from build123d import *

# Parameters (mm, degrees)
F0_R     = 4.05
F1_DEPTH = 1.5
F2_R     = 1
F3_DEPTH = 12.5


with BuildPart() as f1:
    # F0 (on Front) → F1 (new body, symmetric)
    with BuildSketch(Plane.XZ):
        with BuildLine():
            Line((0.714422, -9.773925), (32.096751, -7.480044))
            ThreePointArc((32.096751, -7.480044), (39.05, 0), (32.096751, 7.480044))
            Line((32.096751, 7.480044), (0.714422, 9.773925))
            ThreePointArc((0.714422, 9.773925), (-9.8, 0), (0.714422, -9.773925))
        make_face()
        Circle(F0_R, mode=Mode.SUBTRACT)
        with BuildLine():
            ThreePointArc((32, 0.95), (32.95, 0), (32, -0.95))
            Line((32, -0.95), (7, -0.95))
            ThreePointArc((7, -0.95), (6.05, 0), (7, 0.95))
            Line((7, 0.95), (32, 0.95))
        make_face(mode=Mode.SUBTRACT)
    extrude(amount=F1_DEPTH, both=True)

    # F2 (on Top) → F3 (cut, symmetric)
    with BuildSketch(Plane.XY):
        Circle(F2_R)
    extrude(amount=F3_DEPTH, both=True, mode=Mode.SUBTRACT)


solid = f1.part
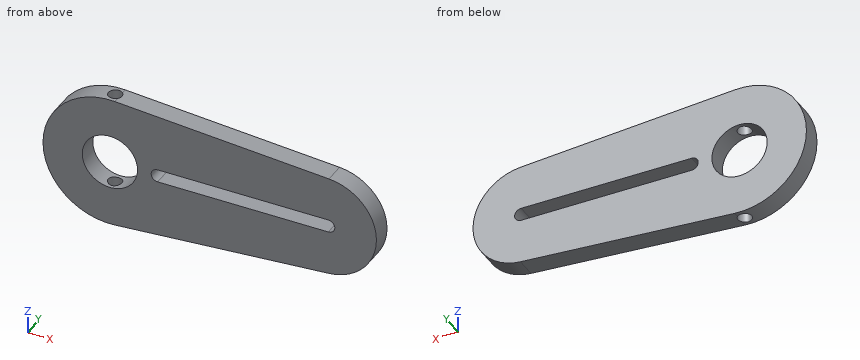
Geometry check sheet. Reference: the model listing, model coordinates, mm. Round coordinates to 2 decimals unless told otherwise and drop trailing zeros. Write each loop counter-clockwise with the first axis right and the second up, starting at its lowest first coordinate (ties: lowest second). Pieces come first, ordered by that corner, then holes.
Item 1: Section check A-A (x = 0). Record the boundary of the cut face in (y, z).
Determined:
outline: (-1.5, -9.8) - (-1, -9.8) - (-1, -4.05) - (-1.5, -4.05) - close; (-1.5, 4.05) - (-1, 4.05) - (-1, 9.8) - (-1.5, 9.8) - close; (1, -9.8) - (1.5, -9.8) - (1.5, -4.05) - (1, -4.05) - close; (1, 4.05) - (1.5, 4.05) - (1.5, 9.8) - (1, 9.8) - close
Item 2: Go/stop test with flat-tipped pins: pin 1 Ø1.2 at (x, y) = (0, 0) entering from -Z; pin 2 Ø1.5 at (x, y) = (29.5, 1) entering from +Z; pin 3 Ø1.5 at (x, y) = (15, 0.5) entering from -Z. Record where each tip stops, or that it passes through.
Determined:
pin 1: passes through
pin 2: stops at z = 7.72
pin 3: stops at z = -8.78
Item 3: Section check D-D (x = 10). Record the boundary of the cut face in (y, z).
Determined:
outline: (-1.5, -9.1) - (1.5, -9.1) - (1.5, -0.95) - (-1.5, -0.95) - close; (-1.5, 0.95) - (1.5, 0.95) - (1.5, 9.1) - (-1.5, 9.1) - close
Item 4: Section check C-C (y = 0). Record the boundary of the cut face in (x, z), plus the area to 3 significant figures.
Determined:
outline: (-1, -9.75) - (-1, -3.92) arc R4.05 cw to (-1, 3.92) - (-1, 9.75) arc R9.8 ccw to start; (1, -9.75) - (32.1, -7.48) arc R7.5 ccw to (32.1, 7.48) - (1, 9.75) - (1, 3.92) arc R4.05 cw to (1, -3.92) - close; hole (7, -0.95) - (32, -0.95) arc R0.95 ccw to (32, 0.95) - (7, 0.95) arc R0.95 ccw to start
area: 662 mm2
Item 5: Section check B-B (z = 0). Record the boundary of the cut face in (x, y), plus the area to 4 significant figures.
Determined:
outline: (-9.8, -1.5) - (-4.05, -1.5) - (-4.05, 1.5) - (-9.8, 1.5) - close; (4.05, -1.5) - (6.05, -1.5) - (6.05, 1.5) - (4.05, 1.5) - close; (32.95, -1.5) - (39.05, -1.5) - (39.05, 1.5) - (32.95, 1.5) - close
area: 41.55 mm2
Item 6: Material ranges on line 1 along Y through (x, z) = (0, -5.45); line 2 along X through (y, z) = (0.1, -2); line 3 along X through (y, z) = (0, 5.6), recorded low to high.
Determined:
line 1: y = -1.5 to -1, 1 to 1.5
line 2: x = -9.59 to -3.52, 3.52 to 38.78
line 3: x = -8.04 to -1, 1 to 36.54
